Study the drawing (mm; zero at the part's minimum x, y, z) and answer. A direction names the side the tool comes from. Round coordinates to 2 decimals unless told otherwise and drop trailing zeros. Write each loop counter-clockwise with the first axis right and the second up, starting at its lowest first coordinate (ties: lowest second). Pieces come first, ordered by that corner, then holes. Notation, with made-up numbers: (-20.75, -30) - (2.25, -30) arc R21 ccw to (2.25, -16) - close; hole circle Ø11 at (6.25, 47). An arc over 180 degrees is marked (long way). Use one line per item in the form item = value. Start each with the question number.
1) The part is cut by section B-B, the plane y = 5.75. Give the vertices of the cut face in (x, z).
2) The part is cut by section D-D, the plane y = 2.25. Give the vertices of the cut face in (x, z).
3) The part is cut by section C-C, the plane z = 2.9. Give the vertices of the cut face in (x, y).
4) Consider line 1 along X through (y, z) = (7, 0.55); line 2 along Z through (x, y) = (5.75, 9.5); line 3 along Y through (x, z) = (10, 3.5) (1 decimal). Determine where each line is inside the solid, lowest interval first. Write a range as from..to.
5) For the marked faces 5 and 6, determine the directions among +Z, -Z, +X, -X, +Y, -Y from which every point of the face is accessible in a straight line to the end or side of a thin tool.
6) For a pull along Y with two mould halves and no side action, classify the marked faces 1, 2, 3 and 4 as released by +Y, released by -Y, zero draft, split by the parting line, or undercut.
7) This flat-tipped pin is pushed along its axis until it touches: pin 1 (1.5 mm diameter, centred on x = 2.5, y = 5, fed in from +Z). Where does it stop, or does it pass through?
8) The part is cut by section A-A, the plane x = 7.25. Give the vertices of the cut face in (y, z).
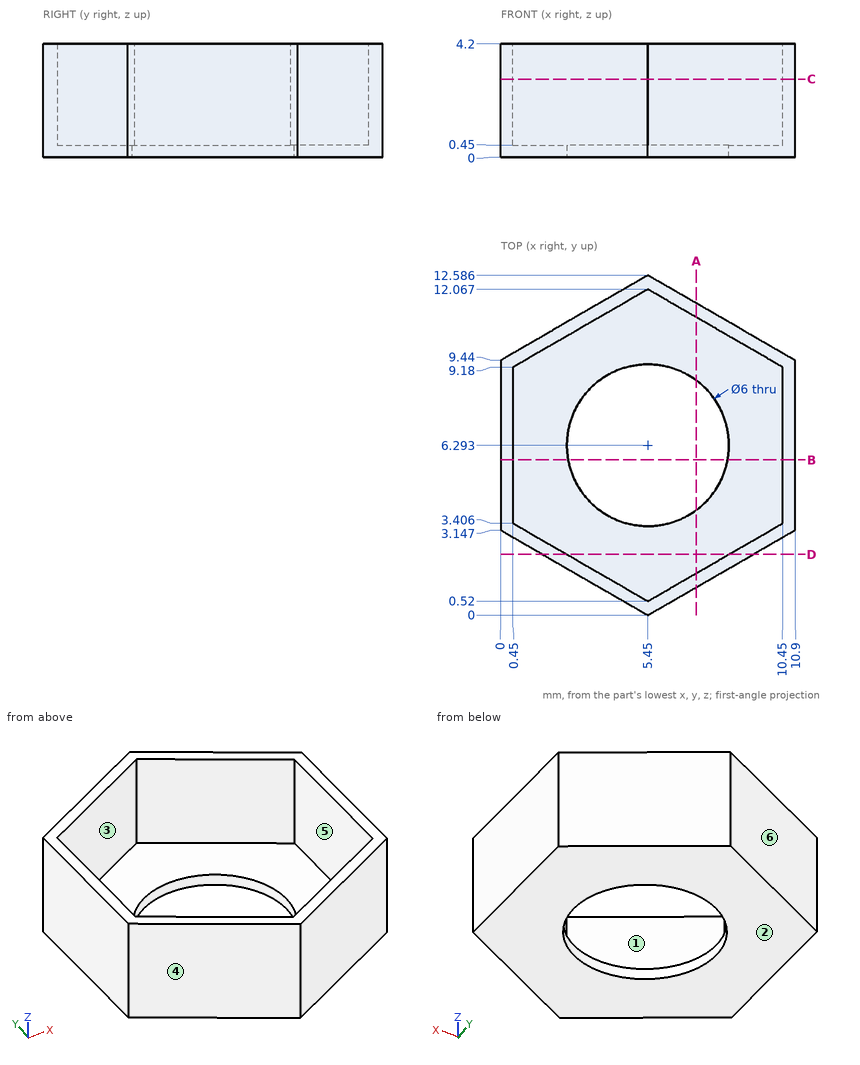
Geometry results:
q1.outline = (0, 0) - (2.5, 0) - (2.5, 0.45) - (0.45, 0.45) - (0.45, 4.2) - (0, 4.2) - close; (8.4, 0) - (10.9, 0) - (10.9, 4.2) - (10.45, 4.2) - (10.45, 0.45) - (8.4, 0.45) - close
q2.outline = (1.55, 0) - (9.35, 0) - (9.35, 4.2) - (8.45, 4.2) - (8.45, 0.45) - (2.45, 0.45) - (2.45, 4.2) - (1.55, 4.2) - close
q3.outline = (0, 3.15) - (5.45, 0) - (10.9, 3.15) - (10.9, 9.44) - (5.45, 12.59) - (0, 9.44) - close; hole (0.45, 3.41) - (5.45, 0.52) - (10.45, 3.41) - (10.45, 9.18) - (5.45, 12.07) - (0.45, 9.18) - close
q4.line_1 = 0..0.45, 10.45..10.9
q4.line_2 = 0..0.45
q4.line_3 = 2.6..3.1, 9.4..10
q5.face_5 = +Z
q5.face_6 = +Z, -Z, -X, +Y
q6.face_1 = undercut
q6.face_2 = zero draft
q6.face_3 = undercut
q6.face_4 = released by -Y
q7.pin_1 = 0.45
q8.outline = (1.04, 0) - (3.89, 0) - (3.89, 0.45) - (1.56, 0.45) - (1.56, 4.2) - (1.04, 4.2) - close; (8.69, 0) - (11.55, 0) - (11.55, 4.2) - (11.03, 4.2) - (11.03, 0.45) - (8.69, 0.45) - close
